Source: three-view drawing plus pictorial views. Frame: mm from the lowest corner of the part. Round coordinates to 2 decimals unless told otherwise and drop trailing zeros. Write each loop counter-clockwise with the first axis right and the second up, starting at its lowest first coordinate (ties: lowest second). Pieces come first, ordered by that corner, then holes. Notation, with made-up numbers: M -34.5,51.25 L -19.5,51.25 A20 ccw -19.5,65.25 Z; hole C 88.5,37 d7. An arc over 180 degrees is marked long. Answer in a Markdown table with one row per item.
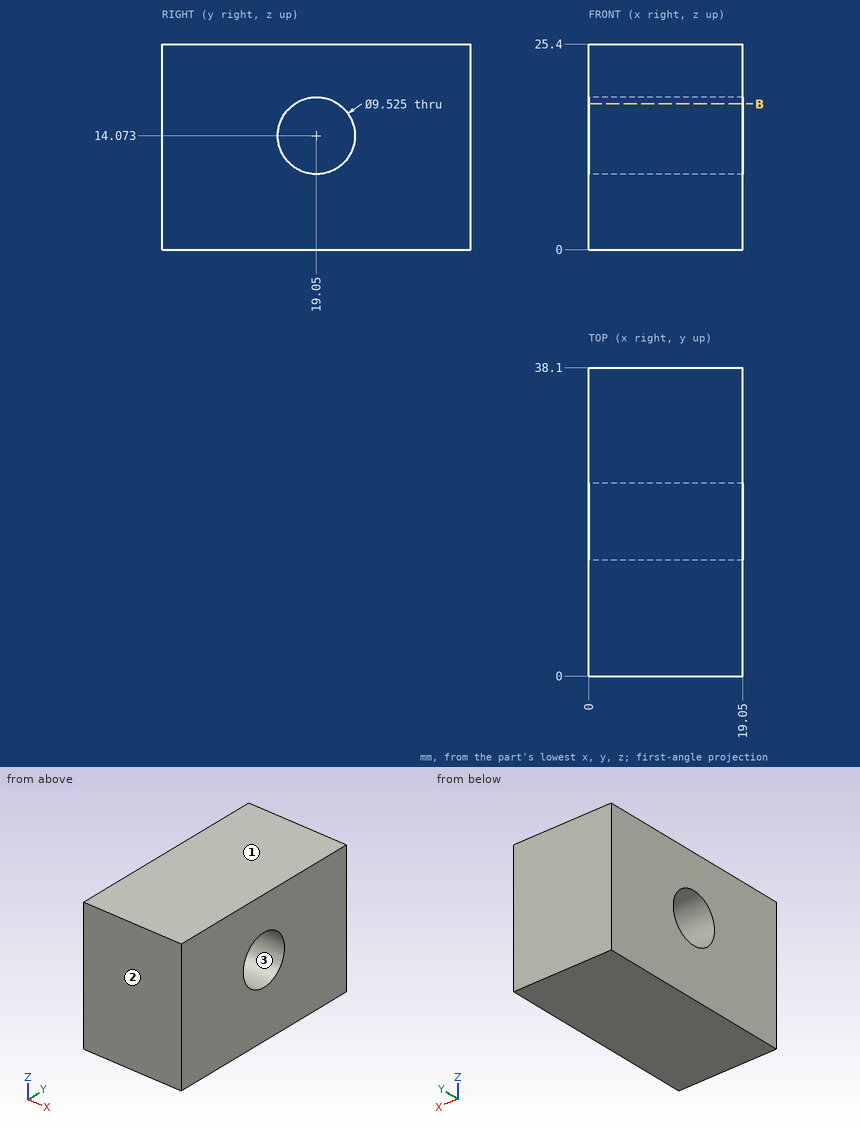
Q1. Section B-B (z = 18). Return loops of the section in (x, y), and give its area (3 significant figures).
Solutions:
| item | result |
|---|---|
| outline | M 0,0 L 19.05,0 L 19.05,16.36 L 0,16.36 Z; M 0,21.74 L 19.05,21.74 L 19.05,38.1 L 0,38.1 Z |
| area | 623 mm2 |
Q2. Pull-direction query (Z, two-part tool) for the marked faces 1, 2 and 3; classes: pulls with the +Z half, pulls with the -Z half, needs draft (parallel to the pull), parting line crosses it, or undercut.
Solutions:
| item | result |
|---|---|
| face 1 | pulls with the +Z half |
| face 2 | needs draft |
| face 3 | undercut |
Q3. Material intervals for probe 1 along Z at (x, y) = (13.25, 19.05) (1 decimal); probe 2 along Y at (x, z) = (15.75, 14.25); probe 3 along Y at (x, z) = (3.75, 11), sorted ascending.
Solutions:
| item | result |
|---|---|
| probe 1 | z = 0 to 9.3, 18.8 to 25.4 |
| probe 2 | y = 0 to 14.29, 23.81 to 38.1 |
| probe 3 | y = 0 to 15.41, 22.69 to 38.1 |
Q4. Contact query for flat-ended pins moving along their axis: pin 1 Ø5 at (x, z) = (13.5, 10) entering from -Y; pin 2 Ø8.5 at (y, z) = (19.05, 14.07) entering from +X. Output: stop coordinate, or through.
Solutions:
| item | result |
|---|---|
| pin 1 | stops at y = 0 |
| pin 2 | passes through |
